Study the drawing (mm; zero at the part's minimum x, y, z) and answer. A direction names the side the tool comes from. Coordinates: 2 decimals unless noted, no trailing zeros. Loops run counter-clockwise (first coordinate to the right, second up) from the corner with the lowest first, then second, coordinate; pieces in that order, holes last. Notation, with made-up numbers: (-20.5, -11.75) -> (23.5, -11.75) arc R9 cw to (23.5, -3.75) -> close; hole circle Ø1 at (58.5, 13). An arc over 180 degrees is marked (long way). Answer as a JSON object with one key per item and string values. Group by question number.
Q1. Each of these flat-tipped pins is pushed along its axis until it touches: P1, Ø2.5, axis at x = 9.85, y = 2.04, coming from the +Z side; P2, Ø4.5, axis at x = 42.5, y = 1.5, coming from the +Z side; P3, Ø6, axis at x = 44, z = 13, coming from the -Y side; P4, Ø4.5, axis at x = 43.5, z = 12, coming from the +Y side. Where does it stop, or does it pass through?
Q2. The part is cut by section B-B on y = 5.25. Write down the section's boundary in (x, z).
Q3. The part is cut by section D-D on y = 1.5. Write down the section's boundary in (x, z).
Q4. Straight lines are drawn through the part: line 1 along Y through (x, z) = (22, 9); line 2 along X through (y, z) = (22.5, 6.75); line 3 along X through (y, z) = (20, 10). For each, find the intervals that lie inside material, in ascending order. Write a range as [from, to].
Q5. Determine the mould class of the marked faces 1, 2 and 3 for opening direction Y: released by +Y, released by -Y, zero draft, split by the parting line, or undercut.
Q6. The part is cut by section A-A on z = 4.5. Write down the section's boundary in (x, y), and give its area (3 significant figures).
Q7. For the marked faces 4, 5, 6, 7 and 8, determine the directions among +Z, -Z, +X, -X, +Y, -Y from which every point of the face is accessible in a straight line to the end or side of a thin tool.
Q8. The part is cut by section C-C on x = 5. Write down the section's boundary in (y, z), and give its area (3 significant figures).
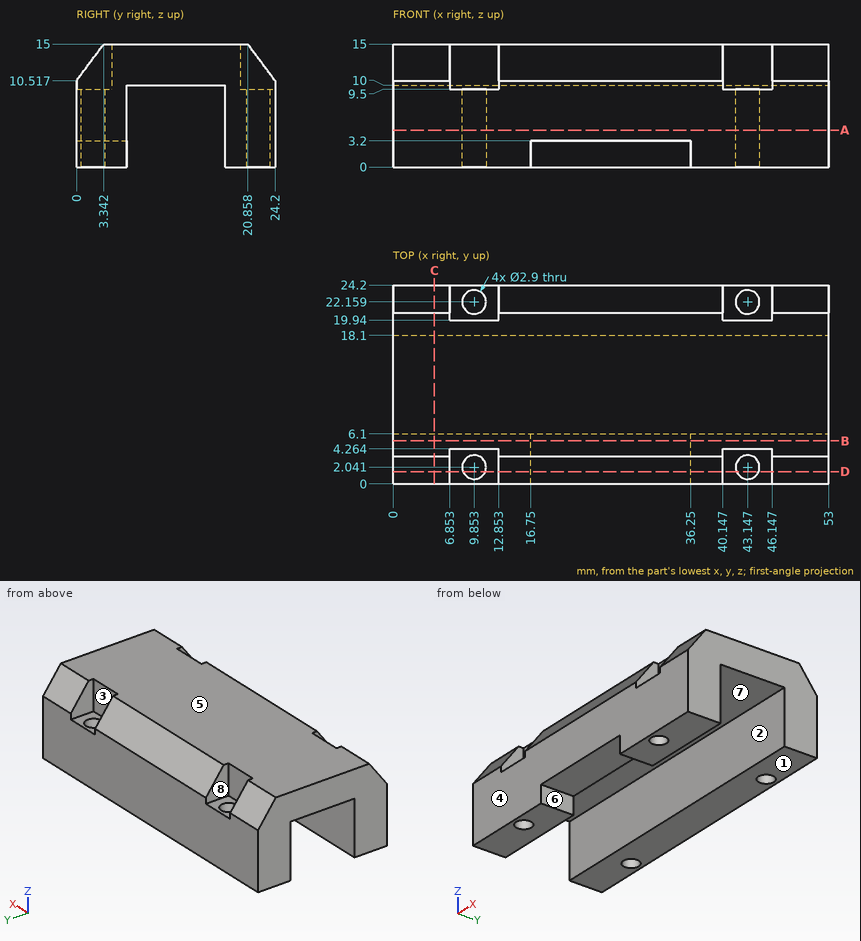
Final values:
{
 "1": {"P1": "passes through", "P2": "stops at z = 9.5", "P3": "stops at y = 0.29", "P4": "stops at y = 19.94"},
 "2": {"outline": "(0, 0) -> (16.75, 0) -> (16.75, 3.2) -> (36.25, 3.2) -> (36.25, 0) -> (53, 0) -> (53, 15) -> (0, 15) -> close"},
 "3": {"outline": "(0, 0) -> (8.51, 0) -> (8.51, 9.5) -> (6.85, 9.5) -> (6.85, 12.53) -> (0, 12.53) -> close; (11.2, 0) -> (16.75, 0) -> (16.75, 3.2) -> (36.25, 3.2) -> (36.25, 0) -> (41.8, 0) -> (41.8, 9.5) -> (40.15, 9.5) -> (40.15, 12.53) -> (12.85, 12.53) -> (12.85, 9.5) -> (11.2, 9.5) -> close; (44.49, 0) -> (53, 0) -> (53, 12.53) -> (46.15, 12.53) -> (46.15, 9.5) -> (44.49, 9.5) -> close"},
 "4": {"line 1": "y = [0, 6.1], [18.1, 24.2]", "line 2": "x = [0, 8.44], [11.26, 41.74], [44.56, 53]", "line 3": "x = [0, 6.85], [12.85, 40.15], [46.15, 53]"},
 "5": {"face 1": "zero draft", "face 2": "undercut", "face 3": "released by +Y"},
 "6": {"outline": "(0, 0) -> (53, 0) -> (53, 6.1) -> (0, 6.1) -> close; (0, 18.1) -> (53, 18.1) -> (53, 24.2) -> (0, 24.2) -> close; hole circle Ø2.9 at (9.85, 2.04); hole circle Ø2.9 at (9.85, 22.16); hole circle Ø2.9 at (43.15, 2.04); hole circle Ø2.9 at (43.15, 22.16)", "area": "620 mm2"},
 "7": {"face 4": "+Z, -Z, +X, -X, -Y", "face 5": "+Z, +X, -X, +Y, -Y", "face 6": "-Z, -Y", "face 7": "-Z, +X, -X", "face 8": "+Z, +Y"},
 "8": {"outline": "(0, 0) -> (6.1, 0) -> (6.1, 10) -> (18.1, 10) -> (18.1, 0) -> (24.2, 0) -> (24.2, 10.52) -> (20.86, 15) -> (3.34, 15) -> (0, 10.52) -> close", "area": "228 mm2"}
}
